from build123d import *

# Parameters (mm, degrees)
ESQUISSE3_W             = 75
ESQUISSE3_H             = 60
BOSS_EXTRU_4_DEPTH      = 2
ESQUISSE7_R             = 3
ESQUISSE7_R_2           = 1
ENL_V_MAT_EXTRU_1_DEPTH = 2
ESQUISSE9_R             = 3
BOSS_EXTRU_5_DEPTH      = 40


with BuildPart() as part:
    # Esquisse3 → Boss.-Extru.4 (new body)
    with BuildSketch(Plane.XY):
        Rectangle(ESQUISSE3_W, ESQUISSE3_H)
    extrude(amount=BOSS_EXTRU_4_DEPTH)

    # Esquisse7 → Enlèv. mat.-Extru.1 (cut)
    with BuildSketch(Plane.XY.offset(2)):
        with Locations((-17, 13.6)):
            Circle(ESQUISSE7_R)
        with Locations((17, 13.6)):
            Circle(ESQUISSE7_R)
        with Locations((7.649218941, -7.4)):
            Circle(ESQUISSE7_R_2)
    extrude(amount=-ENL_V_MAT_EXTRU_1_DEPTH, mode=Mode.SUBTRACT)

    # Esquisse9 → Boss.-Extru.5 (add)
    with BuildSketch(Plane.XY.offset(2)):
        with Locations((-34.10132307, 26.617640071)):
            Circle(ESQUISSE9_R)
        with Locations((33.292276259, 26.617640071)):
            Circle(ESQUISSE9_R)
        with Locations((33.292276259, -26.213116666)):
            Circle(ESQUISSE9_R)
        with Locations((-34.10132307, -26.213116666)):
            Circle(ESQUISSE9_R)
    extrude(amount=BOSS_EXTRU_5_DEPTH)


solid = part.part
For this review, take the finished solid that the model builds, in its own axes (mm). A direction names the side the tool comes from. Coordinates: 2 decimals unless noted, no trailing zeros. Order: outer loops, then holes, each group sorted by start corner. A loop starts at its lowest first (then second) coordinate and runs counter-clockwise, first axis right, second up. Notation, with made-up numbers: (-26.75, 11.25) - (-1.75, 11.25) arc R24 ccw to (-1.75, 30.25) - close; hole circle Ø4 at (-11, -35). An arc over 180 degrees is marked (long way). Use one line per item in the form item = value.
Q1. For probe 1 along Y at (x, z) = (-17, 1.1); probe 2 along Z at (x, y) = (5.5, -26.5); probe 3 along Y at (x, z) = (-32.5, 34), list the stretches that pass through material, from the lowest coordinate up. Write a range as from..to.
Checked values:
probe_1 = -30..10.6, 16.6..30
probe_2 = 0..2
probe_3 = -28.75..-23.68, 24.08..29.15
Q2. Draft analysis for pull direction Y (two halves, no side actions). For faces 3 (the flat face through (-1, 30, 1)), 4 (the flat face through (-34, -26, 42)), 5 (the flat face through (-1, -30, 1)), 6 (the cylindrical face through (7.52, -6.41, 1.01)), state which applies: +Y half, -Y half, draft (parallel to the pull), parting line (faces both ways), or undercut.
Checked values:
face_3 = +Y half
face_4 = draft
face_5 = -Y half
face_6 = undercut
Q3. For faces 1 (the cylindrical face through (36.064, -27.362, 21.72)), 2 (the flat face through (33, -26, 42)), list the 3-axis set-ups (+Z, -Z, +X, -X, +Y, -Y) from which the entire face can be reached by the end or side of a thin tool; tool diameter is ignored.
Checked values:
face_1 = +Z
face_2 = +Z, +X, -X, +Y, -Y
Q4. Consider section C-C (y = -7.4). Give the boundary of the cut face in (x, z).
Checked values:
outline = (-37.5, 0) - (6.65, 0) - (6.65, 2) - (-37.5, 2) - close; (8.65, 0) - (37.5, 0) - (37.5, 2) - (8.65, 2) - close
Q5. Consider section B-B (x = -17). Give the boundary of the cut face in (y, z).
Checked values:
outline = (-30, 0) - (10.6, 0) - (10.6, 2) - (-30, 2) - close; (16.6, 0) - (30, 0) - (30, 2) - (16.6, 2) - close
Q6. For P1, Ø10, axis at x = -16, y = 11, coming from the +Z side, flat-tipped, find the tip position at first contact; note if it passes through.
Checked values:
P1 = 2
Q7. Consider section D-D (z = 39). Give the boundary of the cut face in (x, y).
Checked values:
outline = circle Ø6 at (-34.1, -26.21); circle Ø6 at (-34.1, 26.62); circle Ø6 at (33.29, -26.21); circle Ø6 at (33.29, 26.62)
Q8. Consider section A-A (y = 13.6). Give the boundary of the cut face in (x, z), then the cut area to 3 significant figures.
Checked values:
outline = (-37.5, 0) - (-20, 0) - (-20, 2) - (-37.5, 2) - close; (-14, 0) - (14, 0) - (14, 2) - (-14, 2) - close; (20, 0) - (37.5, 0) - (37.5, 2) - (20, 2) - close
area = 126 mm2
